Geometry: final body of the model. Coordinates: model frame, mm. Face numbers are marked on the shaded views. A direction names the side the tool comes from. Give positions to 0.01 mm unless a question says otherwise; leave off trailing zeros. Write each loop counter-clockwise with the first axis right and the second up, starting at its lowest first coordinate (ties: lowest second). Pieces come first, ordered by that corner, then holes. Notation, with made-up numbers: M -26.75,5.25 L 23.25,5.25 A19 ccw 23.25,11.25 Z; hole C 38.25,36 d5. An arc over 180 degrees is marked long. Use a Markdown table: item, result. Add a question column.
(1) Reachability of the marked faces 1, 2 and 3 from +Z, -Z, +X, -X, +Y, -Y: full face, straight path, thin tool, end or side. Return the list, or none.
(2) Cut plane B-B (y = 8). Output: boundary loops of the cut face in (x, z), plus the area to 3 significant figures.
(3) Cut plane C-C (y = -33). Output: boundary loops of the cut face in (x, z).
(4) Draft query along Z for the marked faces 4, 5, 6 and 7. Return one class per face: released by +Z, released by -Z, zero draft, split by the parting line, or undercut.
(5) Pin query (flat end, axial travel): pin 1 Ø15 at (x, z) = (6.5, 33.5) entering from -Y; pin 2 Ø2 at (y, z) = (1.5, 24) entering from +X; pin 3 Ø6 at (x, z) = (19.5, 32) entering from +Y; pin 4 Ø5 at (x, y) = (28.5, 29) entering from -Z (3 decimals). Return the tip coordinate at first contact, or that it passes through.
(6) Cut plane A-A (x = 0). Output: boundary loops of the cut face in (y, z), plus the area to 3 significant figures.
(7) Material intervals for L1, parallel to Z at x = -21.5, y = 16; L2, parallel to Z at x = -24, y = -21.5; L3, parallel to Y at x = -12, z = 40, sorted ascending.
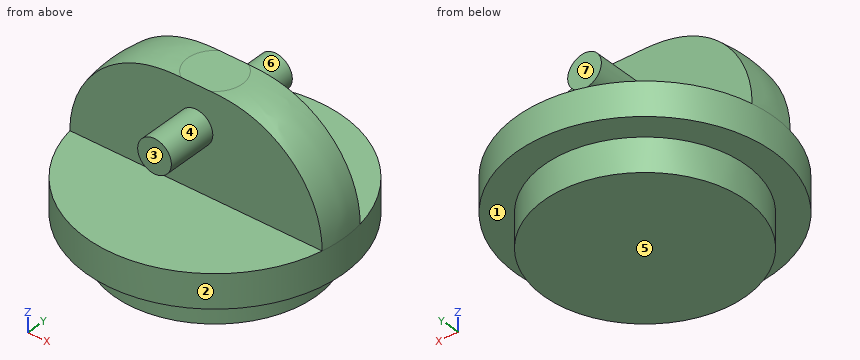
```python
from build123d import *

# Parameters (mm, degrees)
F0_R        = 30
F1_DEPTH    = 10
F2_R        = 38.1255
F2_R_2      = 30
F3_DEPTH    = 10
F5_DEPTH    = 10
F7_DEPTH    = 20
F8_T2_ANGLE = 246.2138015041
F8_T4_ANGLE = 246.2138015041
F10_R       = 5
F11_DEPTH   = 15
F9_R        = 5
F12_DEPTH   = 15


# Not quite as in the source:
# - a fillet or chamfer that OpenCascade refuses, or shapes differently, is made with other operations: its cross-section is extruded or revolved along the edge and cut away or added


with BuildPart() as f1:
    # F0 (on Top) → F1 (new body)
    with BuildSketch(Plane.XY):
        Circle(F0_R)
    extrude(amount=F1_DEPTH)

    # F2 (on face) → F3 (join)
    with BuildSketch(Plane.XY.offset(10)):
        Circle(F2_R)
        Circle(F2_R_2, mode=Mode.SUBTRACT)
        Circle(F2_R_2)
    extrude(amount=F3_DEPTH)

    # F4 (on face) → F5 (join)
    with BuildSketch(Plane.XY.offset(20)):
        with BuildLine():
            Line((37.5, 6.8777721865), (-37.5, 6.8777721865))
            ThreePointArc((-37.5, 6.8777721865), (-38.1255, 0), (-37.5, -6.8777721865))
            Line((-37.5, -6.8777721865), (37.5, -6.8777721865))
            ThreePointArc((37.5, -6.8777721865), (37.9688029851, -3.4530783549), (38.1255, 0))
            ThreePointArc((38.1255, 0), (37.9688029851, 3.4530783549), (37.5, 6.8777721865))
        make_face()
    extrude(amount=F5_DEPTH)

    # F6 (on face) → F7 (join)
    with BuildSketch(Plane.XY.offset(30)):
        with BuildLine():
            Line((37.5, 6.8777721865), (-37.5, 6.8777721865))
            ThreePointArc((-37.5, 6.8777721865), (-38.1255, 0), (-37.5, -6.8777721865))
            Line((-37.5, -6.8777721865), (37.5, -6.8777721865))
            ThreePointArc((37.5, -6.8777721865), (38.1255, 0), (37.5, 6.8777721865))
        make_face()
    extrude(amount=F7_DEPTH)

    # F8: fillet of radius 30 on 2 edges, made by hand

    # F8_s1 → F8_t2 (revolve, cut)
    with BuildSketch(Plane(origin=(0, 0, 0), x_dir=(0, 0, 1), z_dir=(-0.8376529376, 0.5462028526, 0))):
        with BuildLine():
            ThreePointArc((20, -38.1255), (41.2132034356, -29.3387034356), (50, -8.1255))
            Line((50, -8.1255), (50, -38.1255))
            Line((50, -38.1255), (20, -38.1255))
        make_face()
    revolve(axis=Axis((0, 0, 50), (0, 0, 1)), revolution_arc=F8_T2_ANGLE, mode=Mode.SUBTRACT)

    # F8_s3 → F8_t4 (revolve, cut)
    with BuildSketch(Plane(origin=(0, 0, 0), x_dir=(0, 0, 1), z_dir=(0.8376529376, -0.5462028526, 0))):
        with BuildLine():
            ThreePointArc((20, -38.1255), (41.2132034356, -29.3387034356), (50, -8.1255))
            Line((50, -8.1255), (50, -38.1255))
            Line((50, -38.1255), (20, -38.1255))
        make_face()
    revolve(axis=Axis((0, 0, 50), (0, 0, 1)), revolution_arc=F8_T4_ANGLE, mode=Mode.SUBTRACT)

    # F10 (on face) → F11 (join)
    with BuildSketch(Plane(origin=(0, 6.8777721865, 0), x_dir=(-1, 0, 0), z_dir=(0, 1, 0))):
        with Locations((0, 38)):
            Circle(F10_R)
    extrude(amount=F11_DEPTH)

    # F9 (on face) → F12 (join)
    with BuildSketch(Plane.XZ.offset(6.8777721865)):
        with Locations((0, 38)):
            Circle(F9_R)
    extrude(amount=F12_DEPTH)


solid = f1.part
```
Answer list:
| question | item | result |
|---|---|---|
| 1 | face 1 | -Z |
| 1 | face 2 | +Z, -Z |
| 1 | face 3 | +Z, +X, -X, -Y |
| 2 | outline | M -37.28,10 L -28.91,10 L -28.91,0 L 28.91,0 L 28.91,10 L 37.28,10 L 37.28,20 L -37.28,20 Z; C 0,38 d10 |
| 2 | area | 1,400 mm² |
| 3 | outline | M -19.09,10 L 19.09,10 L 19.09,20 L -19.09,20 Z |
| 4 | face 4 | undercut |
| 4 | face 5 | released by -Z |
| 4 | face 6 | undercut |
| 4 | face 7 | zero draft |
| 5 | pin 1 | y = -21.88 |
| 5 | pin 2 | x = 37.95 |
| 5 | pin 3 | y = 6.88 |
| 5 | pin 4 | through |
| 6 | outline | M -38.13,10 L -30,10 L -30,0 L 30,0 L 30,10 L 38.13,10 L 38.13,20 L 6.88,20 L 6.88,33 L 21.88,33 L 21.88,43 L 6.88,43 L 6.88,50 L -6.88,50 L -6.88,43 L -21.88,43 L -21.88,33 L -6.88,33 L -6.88,20 L -38.13,20 Z |
| 6 | area | 2,080 mm² |
| 7 | L1 | 0 to 20 |
| 7 | L2 | 10 to 20 |
| 7 | L3 | -6.88 to 6.88 |
